```python
from build123d import *

# Parameters (mm, degrees)
SKETCH1_R           = 40
SKETCH1_R_2         = 9.5
SKETCH1_R_3         = 2.5
BOSS_EXTRUDE2_DEPTH = 8
SKETCH3_R           = 1.5
CUT_EXTRUDE1_DEPTH  = 8
SKETCH4_R           = 7
SKETCH4_R_2         = 5
BOSS_EXTRUDE6_DEPTH = 20


with BuildPart() as part:
    # Sketch1 → Boss-Extrude2 (new body)
    # profile 1 of 2: a face of its own
    with BuildSketch(Plane(origin=(0, 0, 0), x_dir=(1, 0, 0), z_dir=(0, 1, 0))):
        with BuildLine():
            Line((-44, 22), (-44, -22))
            Line((-44, -22), (-33.406586177, -22))
            ThreePointArc((-33.406586177, -22), (-40, 0), (-33.406586177, 22))
            Line((-33.406586177, 22), (-44, 22))
        make_face()
    # profile 2 of 2: a face of its own
    with BuildSketch(Plane(origin=(0, 0, 0), x_dir=(1, 0, 0), z_dir=(0, 1, 0))):
        Circle(SKETCH1_R)
        with Locations(Location((-22, 0, 0), (0, 0, 270))):
            Circle(SKETCH1_R_2, mode=Mode.SUBTRACT)
        with Locations(Location((11, 32.25, 0), (0, 0, 270))):
            Circle(SKETCH1_R_3, mode=Mode.SUBTRACT)
        with Locations(Location((-11, 32.25, 0), (0, 0, 270))):
            Circle(SKETCH1_R_3, mode=Mode.SUBTRACT)
        with Locations(Location((11, -32.25, 0), (0, 0, 270))):
            Circle(SKETCH1_R_3, mode=Mode.SUBTRACT)
        with Locations(Location((-11, -32.25, 0), (0, 0, 270))):
            Circle(SKETCH1_R_3, mode=Mode.SUBTRACT)
        with Locations(Location((32.25, -11, 0), (0, 0, 270))):
            Circle(SKETCH1_R_3, mode=Mode.SUBTRACT)
        with Locations(Location((32.25, 11, 0), (0, 0, 270))):
            Circle(SKETCH1_R_3, mode=Mode.SUBTRACT)
    extrude(amount=BOSS_EXTRUDE2_DEPTH)

    # Sketch3 → Cut-Extrude1 (cut)
    with BuildSketch(Plane(origin=(0, 8, 0), x_dir=(1, 0, 0), z_dir=(0, 1, 0))):
        with Locations(Location((-37.5, 15.5, 0), (0, 0, 270))):
            Circle(SKETCH3_R)
        with Locations(Location((-6.5, 15.5, 0), (0, 0, 270))):
            Circle(SKETCH3_R)
        with Locations(Location((-6.5, -15.5, 0), (0, 0, 270))):
            Circle(SKETCH3_R)
        with Locations(Location((-37.5, -15.5, 0), (0, 0, 270))):
            Circle(SKETCH3_R)
    extrude(amount=-CUT_EXTRUDE1_DEPTH, mode=Mode.SUBTRACT)

    # Sketch4 → Boss-Extrude6 (add)
    # profile 1 of 16: a face of its own
    with BuildSketch(Plane(origin=(0, 8, 0), x_dir=(1, 0, 0), z_dir=(0, 1, 0))):
        with Locations((-21, -21)):
            Circle(SKETCH4_R)
        with Locations(Location((-21, -21, 0), (0, 0, 270))):
            Circle(SKETCH4_R_2, mode=Mode.SUBTRACT)
    # profile 2 of 16: a face of its own
    with BuildSketch(Plane(origin=(0, 8, 0), x_dir=(1, 0, 0), z_dir=(0, 1, 0))):
        with BuildLine():
            ThreePointArc((-16.050252532, -25.949747468), (-25.949747468, -25.949747468), (-25.949747468, -16.050252532))
            Line((-25.949747468, -16.050252532), (-30.640212626, -20.740717689))
            ThreePointArc((-30.640212626, -20.740717689), (-26.162950904, -26.162950904), (-20.740717689, -30.640212626))
            Line((-20.740717689, -30.640212626), (-16.050252532, -25.949747468))
        make_face()
    # profile 3 of 16: a face of its own
    with BuildSketch(Plane(origin=(0, 8, 0), x_dir=(1, 0, 0), z_dir=(0, 1, 0))):
        with BuildLine():
            Line((-14.67544468, -18), (0, -3.32455532))
            Line((0, -3.32455532), (-3.32455532, 0))
            Line((-3.32455532, 0), (-18, -14.67544468))
            ThreePointArc((-18, -14.67544468), (-16.050252532, -16.050252532), (-14.67544468, -18))
        make_face()
    # profile 4 of 16: a face of its own
    with BuildSketch(Plane(origin=(0, 8, 0), x_dir=(1, 0, 0), z_dir=(0, 1, 0))):
        with BuildLine():
            ThreePointArc((14.67544468, -24), (14, -21), (14.67544468, -18))
            Line((14.67544468, -18), (14, -18))
            Line((14, -18), (-14.67544468, -18))
            ThreePointArc((-14.67544468, -18), (-14.170948556, -19.462451178), (-14, -21))
            ThreePointArc((-14, -21), (-14.170948556, -22.537548822), (-14.67544468, -24))
            Line((-14.67544468, -24), (14, -24))
            Line((14, -24), (14.67544468, -24))
        make_face()
    # profile 5 of 16: a face of its own
    with BuildSketch(Plane(origin=(0, 8, 0), x_dir=(1, 0, 0), z_dir=(0, 1, 0))):
        with Locations((21, -21)):
            Circle(SKETCH4_R)
        with Locations(Location((21, -21, 0), (0, 0, 270))):
            Circle(SKETCH4_R_2, mode=Mode.SUBTRACT)
    # profile 6 of 16: a face of its own
    with BuildSketch(Plane(origin=(0, 8, 0), x_dir=(1, 0, 0), z_dir=(0, 1, 0))):
        with BuildLine():
            Line((30.640212626, -20.740717689), (25.949747468, -16.050252532))
            ThreePointArc((25.949747468, -16.050252532), (27.467156728, -18.321215973), (28, -21))
            ThreePointArc((28, -21), (23.678784027, -27.467156728), (16.050252532, -25.949747468))
            Line((16.050252532, -25.949747468), (20.740717689, -30.640212626))
            ThreePointArc((20.740717689, -30.640212626), (26.162950904, -26.162950904), (30.640212626, -20.740717689))
        make_face()
    # profile 7 of 16: a face of its own
    with BuildSketch(Plane(origin=(0, 8, 0), x_dir=(1, 0, 0), z_dir=(0, 1, 0))):
        with BuildLine():
            ThreePointArc((14.67544468, -18), (16.050252532, -16.050252532), (18, -14.67544468))
            Line((18, -14.67544468), (3.32455532, 0))
            Line((3.32455532, 0), (0, -3.32455532))
            Line((0, -3.32455532), (14.67544468, -18))
        make_face()
    # profile 8 of 16: a face of its own
    with BuildSketch(Plane(origin=(0, 8, 0), x_dir=(1, 0, 0), z_dir=(0, 1, 0))):
        with BuildLine():
            Line((24, -14.446329174), (24, 14))
            Line((24, 14), (24, 14.67544468))
            ThreePointArc((24, 14.67544468), (21, 14), (18, 14.67544468))
            Line((18, 14.67544468), (18, 14))
            Line((18, 14), (18, -14.111462488))
            Line((18, -14.111462488), (18, -14.67544468))
            ThreePointArc((18, -14.67544468), (21, -14), (24, -14.67544468))
            Line((24, -14.67544468), (24, -14.446329174))
        make_face()
    # profile 9 of 16: a face of its own
    with BuildSketch(Plane(origin=(0, 8, 0), x_dir=(1, 0, 0), z_dir=(0, 1, 0))):
        with BuildLine():
            Line((3.32455532, 0), (18, 14.67544468))
            ThreePointArc((18, 14.67544468), (16.050252532, 16.050252532), (14.67544468, 18))
            Line((14.67544468, 18), (0, 3.32455532))
            Line((0, 3.32455532), (3.32455532, 0))
        make_face()
    # profile 10 of 16: a face of its own
    with BuildSketch(Plane(origin=(0, 8, 0), x_dir=(1, 0, 0), z_dir=(0, 1, 0))):
        Polygon((0, -3.32455532), (3.32455532, 0), (0, 3.32455532), (-3.32455532, 0), align=None)
    # profile 11 of 16: a face of its own
    with BuildSketch(Plane(origin=(0, 8, 0), x_dir=(1, 0, 0), z_dir=(0, 1, 0))):
        with BuildLine():
            Line((-3.32455532, 0), (0, 3.32455532))
            Line((0, 3.32455532), (-14.67544468, 18))
            ThreePointArc((-14.67544468, 18), (-16.050252532, 16.050252532), (-18, 14.67544468))
            Line((-18, 14.67544468), (-3.32455532, 0))
        make_face()
    # profile 12 of 16: a face of its own
    with BuildSketch(Plane(origin=(0, 8, 0), x_dir=(1, 0, 0), z_dir=(0, 1, 0))):
        with BuildLine():
            Line((13.75, 18), (14.67544468, 18))
            ThreePointArc((14.67544468, 18), (14, 21), (14.67544468, 24))
            Line((14.67544468, 24), (-13, 24))
            Line((-13, 24), (-13.890574763, 24))
            Line((-13.890574763, 24), (-14.67544468, 24))
            ThreePointArc((-14.67544468, 24), (-14.170948556, 22.537548822), (-14, 21))
            ThreePointArc((-14, 21), (-14.170948556, 19.462451178), (-14.67544468, 18))
            Line((-14.67544468, 18), (-14.243300619, 18))
            Line((-14.243300619, 18), (13.75, 18))
        make_face()
    # profile 13 of 16: a face of its own
    with BuildSketch(Plane(origin=(0, 8, 0), x_dir=(1, 0, 0), z_dir=(0, 1, 0))):
        with Locations((21, 21)):
            Circle(SKETCH4_R)
        with Locations(Location((21, 21, 0), (0, 0, 270))):
            Circle(SKETCH4_R_2, mode=Mode.SUBTRACT)
    # profile 14 of 16: a face of its own
    with BuildSketch(Plane(origin=(0, 8, 0), x_dir=(1, 0, 0), z_dir=(0, 1, 0))):
        with BuildLine():
            ThreePointArc((28, 21), (27.467156728, 18.321215973), (25.949747468, 16.050252532))
            Line((25.949747468, 16.050252532), (30.640212626, 20.740717689))
            ThreePointArc((30.640212626, 20.740717689), (26.162950904, 26.162950904), (20.740717689, 30.640212626))
            Line((20.740717689, 30.640212626), (16.050252532, 25.949747468))
            ThreePointArc((16.050252532, 25.949747468), (23.678784027, 27.467156728), (28, 21))
        make_face()
    # profile 15 of 16: a face of its own
    with BuildSketch(Plane(origin=(0, 8, 0), x_dir=(1, 0, 0), z_dir=(0, 1, 0))):
        with BuildLine():
            Line((-16.050252532, 25.949747468), (-20.740717689, 30.640212626))
            ThreePointArc((-20.740717689, 30.640212626), (-26.162950904, 26.162950904), (-30.640212626, 20.740717689))
            Line((-30.640212626, 20.740717689), (-25.949747469, 16.050252532))
            ThreePointArc((-25.949747469, 16.050252532), (-25.949747469, 25.949747468), (-16.050252532, 25.949747468))
        make_face()
    # profile 16 of 16: a face of its own
    with BuildSketch(Plane(origin=(0, 8, 0), x_dir=(1, 0, 0), z_dir=(0, 1, 0))):
        with Locations((-21, 21)):
            Circle(SKETCH4_R)
        with Locations(Location((-21, 21, 0), (0, 0, 270))):
            Circle(SKETCH4_R_2, mode=Mode.SUBTRACT)
    extrude(amount=BOSS_EXTRUDE6_DEPTH)


solid = part.part
```
Can you work these out from the model? Positions are in its coordinate system, mm. A direction names the side the tool comes from. Coordinates: 2 decimals unless noted, no trailing zeros. Loops run counter-clockwise (first coordinate to the right, second up) from the corner with the lowest first, then second, coordinate; pieces in that order, holes last. Notation, with made-up numbers: (16, 4) -> (56, 4) arc R24 cw to (56, 27) -> close; hole circle Ø4 at (52.25, -31). An arc over 180 degrees is marked (long way). Put each result on its own line as item: value. Start each with the question number.
Q1. I'm going to push flat-ended pins straight in: P1, Ø8, axis at x = -21, z = 21, coming from the +Y side; P2, Ø10, axis at x = 5, y = 15.5, coming from the +Z side; P3, Ø10, axis at x = 24.5, z = -18, coming from the -Y side; P4, Ø5, axis at y = 21, z = 8, coming from the -X side. Where does each tip first touch, or does it pass through?
Q2. I want a section at C-C (y = 18.25). Count the separate pieces of the cut face and the enclosed holes in it, plus the area to 3 significant figures.
Q3. I want a section at D-D (z = -32.25). Write out the boundary of the cut face in (x, y), plus the area to 3 significant figures.
Q4. For faces 4 (the face through (25.02, 17.86, -15.27)), 5 (the face through (-21, 8, -21)), 6 (the face through (-6.43, 4.06, 14)), 7 (the face through (-26.093, 17.86, -26.233)), 8 (the face through (15.29, 17.86, -25.05)), which set-ups out of +Z, -Z, +X, -X, +Y, -Y let a thin tool reach every point of the face, with its end or its side?
Q5. I want a section at A-A (z = -11). Write out the boundary of the cut face in (x, y).
Q6. I want a section at B-B (x = -10). Write out the boundary of the cut face in (y, z).
Q7. If I drill on line 1 (X direction, y = 5.25, z = -0.5); line 2 (Z direction, x = 34.5, y = 6); line 3 (X direction, y = 24, z = 13), over which ranges is the centre line in solid material (lowest first)? Write a range as [from, to].
Q8. Thinking about a two-plate mould opening in X: for faces 1 (the face through (16.12, 17.86, 19.92)), 2 (the face through (-26.233, 17.86, 26.093)), 3 (the face through (26.233, 17.86, -26.093)), which applies, pulls with the +X half, pulls with the -X half, needs draft (parallel to the pull), parting line crosses it, or undercut?
Taken from the geometry:
1. P1: stops at y = 8
1. P2: stops at z = 24
1. P3: stops at y = 0
1. P4: stops at x = -13.82
2. separate pieces: 1
2. enclosed holes: 7
2. area: 1,310 mm2
3. outline: (-23.66, 0) -> (-13.5, 0) -> (-13.5, 8) -> (-23.66, 8) -> close; (-8.5, 0) -> (8.5, 0) -> (8.5, 8) -> (-8.5, 8) -> close; (13.5, 0) -> (23.66, 0) -> (23.66, 8) -> (13.5, 8) -> close
3. area: 299 mm2
4. face 4: +X, +Y
4. face 5: +Y
4. face 6: +Y, -Y
4. face 7: -Z, -X, +Y
4. face 8: -Z, +Y
5. outline: (-44, 0) -> (29.75, 0) -> (29.75, 8) -> (24, 8) -> (24, 28) -> (18, 28) -> (18, 8) -> (14.32, 8) -> (14.32, 28) -> (7.68, 28) -> (7.68, 8) -> (-7.68, 8) -> (-7.68, 28) -> (-14.32, 28) -> (-14.32, 8) -> (-44, 8) -> close; (34.75, 0) -> (38.46, 0) -> (38.46, 8) -> (34.75, 8) -> close
6. outline: (0, -38.73) -> (8, -38.73) -> (8, -34.54) -> (0, -34.54) -> close; (0, -29.96) -> (8, -29.96) -> (8, -24) -> (28, -24) -> (28, -18) -> (8, -18) -> (8, -13.32) -> (28, -13.32) -> (28, -6.68) -> (8, -6.68) -> (8, 6.68) -> (28, 6.68) -> (28, 13.32) -> (8, 13.32) -> (8, 18) -> (28, 18) -> (28, 24) -> (8, 24) -> (8, 29.96) -> (0, 29.96) -> close; (0, 34.54) -> (8, 34.54) -> (8, 38.73) -> (0, 38.73) -> close
7. line 1: x = [-44, -31.49], [-12.51, 40]
7. line 2: z = [-20.24, -12.09], [-9.91, 9.91], [12.09, 20.24]
7. line 3: x = [-16.32, -9.68], [9.68, 16.32], [18, 24]
8. face 1: undercut
8. face 2: pulls with the -X half
8. face 3: pulls with the +X half
